Input: part model. Units: mm. Frame: model coordinates. Face numbers are marked on the shaded views. Coordinates: 2 decimals unless noted, no trailing zeros. Write each loop counter-clockwise with the first axis right and the second up, starting at its lowest first coordinate (ties: lowest second). Pieces come first, ordered by that corner, then holes. Notation, with made-up numbers: (20, -36.5) - (24, -36.5) arc R11 ccw to (24, -27.5) - close; hole circle Ø10 at (62.5, 85.25). An arc over 180 degrees is marked (long way). Use CSV: the item, a comma, the result in double quotes.
```python
from build123d import *

# Parameters (mm, degrees)
F0_W     = 44.5
F0_H     = 77.5
F0_W_2   = 40.5
F0_H_2   = 73.5
F0_W_3   = 34.2
F0_H_3   = 33.5
F0_W_4   = 3.2
F0_H_4   = 30.9815835953
F0_W_5   = 3.1855669804
F0_H_5   = 13.9315482229
F0_W_6   = 16.6057739407
F0_H_6   = 6.5
F1_DEPTH = 2
F2_W     = 44.5
F2_H     = 77.5
F2_W_2   = 40.5
F2_H_2   = 73.5
F3_DEPTH = 6
F4_R     = 8.5
F5_DEPTH = 1


with BuildPart() as f1:
    # F0 (on Top) → F1 (new body)
    with BuildSketch(Plane.XY):
        Rectangle(F0_W, F0_H)
        Rectangle(F0_W_2, F0_H_2, mode=Mode.SUBTRACT)
        Rectangle(F0_W_2, F0_H_2)
        with Locations((0, 17.5)):
            Rectangle(F0_W_3, F0_H_3, mode=Mode.SUBTRACT)
        with Locations((0, 17.5)):
            Rectangle(F0_W_3, F0_H_3)
        with Locations((-13.7, 17.9407917976)):
            Rectangle(F0_W_4, F0_H_4, mode=Mode.SUBTRACT)
        with Locations((-5.6343034375, 10.3312116116)):
            Rectangle(F0_W_5, F0_H_5, mode=Mode.SUBTRACT)
        with Locations((0, 22.5)):
            Rectangle(F0_W_6, F0_H_6, mode=Mode.SUBTRACT)
        with Locations((13.7, 17.9407917976)):
            Rectangle(F0_W_4, F0_H_4, mode=Mode.SUBTRACT)
    extrude(amount=-F1_DEPTH)

    # F2 (on face) → F3 (join)
    with BuildSketch(Plane(origin=(0, 0, -2), x_dir=(1, 0, 0), z_dir=(0, 0, -1))):
        Rectangle(F2_W, F2_H)
        Rectangle(F2_W_2, F2_H_2, mode=Mode.SUBTRACT)
    extrude(amount=F3_DEPTH)

    # F4 (on face) → F5 (join)
    with BuildSketch(Plane.XY):
        with Locations((-22.25, 38.75)):
            Circle(F4_R)
        with Locations((22.25, 38.75)):
            Circle(F4_R)
        with Locations((22.25, -38.75)):
            Circle(F4_R)
        with Locations((-22.25, -38.75)):
            Circle(F4_R)
    extrude(amount=-F5_DEPTH)


solid = f1.part
```
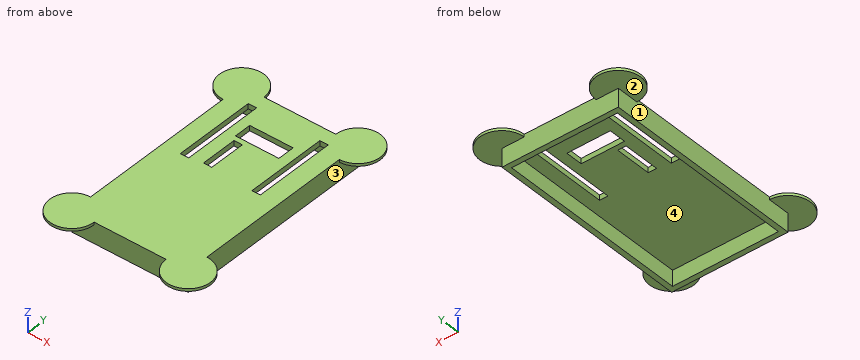
(1) Ray query, probe 1 along Y at (x, z) = (6.5, -6); probe 2 along X at (y, z) = (9, -4.5); probe 3 along X at (y, z) = (-4, -0.75). Return the intervals inside material, ascending. Write a range as from..to.
Check values:
probe 1,"-38.75..-36.75, 36.75..38.75"
probe 2,"-22.25..-20.25, 20.25..22.25"
probe 3,"-22.25..22.25"
(2) Pin query (flat end, axial travel): pin 1 Ø3 at (y, z) = (3, -5) entering from -X; pin 2 Ø4 at (y, z) = (-7.5, -3.5) entering from +X; pin 3 Ø1.5 at (x, y) = (-13.5, -28) entering from -Z. Return the tip coordinate at first contact, or that it passes through.
Check values:
pin 1,"x = -22.25"
pin 2,"x = 22.25"
pin 3,"z = -2"
(3) Cut plane C-C on z = -3.5. Return loops of the section in (x, y).
Check values:
outline,"(-22.25, -38.75) - (22.25, -38.75) - (22.25, 38.75) - (-22.25, 38.75) - close; hole (-20.25, -36.75) - (20.25, -36.75) - (20.25, 36.75) - (-20.25, 36.75) - close"
(4) Cut plane A-A on x = -2. Return loops of the section in (y, z).
Check values:
outline,"(-38.75, -8) - (-36.75, -8) - (-36.75, -2) - (19.25, -2) - (19.25, 0) - (-38.75, 0) - close; (25.75, -2) - (36.75, -2) - (36.75, -8) - (38.75, -8) - (38.75, 0) - (25.75, 0) - close"
(5) Draft query along X for the marked faces 1, 2, 3 and 4. Return one class per face: pulls with the +X half, pulls with the -X half, needs draft (parallel to the pull), parting line crosses it, or undercut.
Check values:
face 1,"pulls with the -X half"
face 2,"needs draft"
face 3,"pulls with the +X half"
face 4,"undercut"
(6) Cut plane B-B on y = 24. Return loops of the section in (x, z).
Check values:
outline,"(-22.25, -8) - (-20.25, -8) - (-20.25, -2) - (-15.3, -2) - (-15.3, 0) - (-22.25, 0) - close; (-12.1, -2) - (-8.3, -2) - (-8.3, 0) - (-12.1, 0) - close; (8.3, -2) - (12.1, -2) - (12.1, 0) - (8.3, 0) - close; (15.3, -2) - (20.25, -2) - (20.25, -8) - (22.25, -8) - (22.25, 0) - (15.3, 0) - close"
(7) Cut plane D-D on y = -6.5. Return loops of the section in (x, z), and give its area (3 significant figures).
Check values:
outline,"(-22.25, -8) - (-20.25, -8) - (-20.25, -2) - (20.25, -2) - (20.25, -8) - (22.25, -8) - (22.25, 0) - (-22.25, 0) - close"
area,"113 mm^2"
